The drawing under review shows one solid part. Ordinate dimensions are in mm from its lowest x, y, z. A direction names the side the tool comes from. Coordinates: 2 decimals unless noted, no trailing zeros. Write each loop counter-clockwise with the first axis right and the second up, starting at its lowest first coordinate (ties: lowest second). Pieces come first, ordered by that corner, then holes. Notation, with made-up numbers: (-30.75, 20) -> (-7.75, 20) arc R10 cw to (-7.75, 27) -> close; hole circle Ø7 at (40, 58). An arc over 180 degrees is marked (long way). Put each result on its own line as item: value. Start each with the question number.
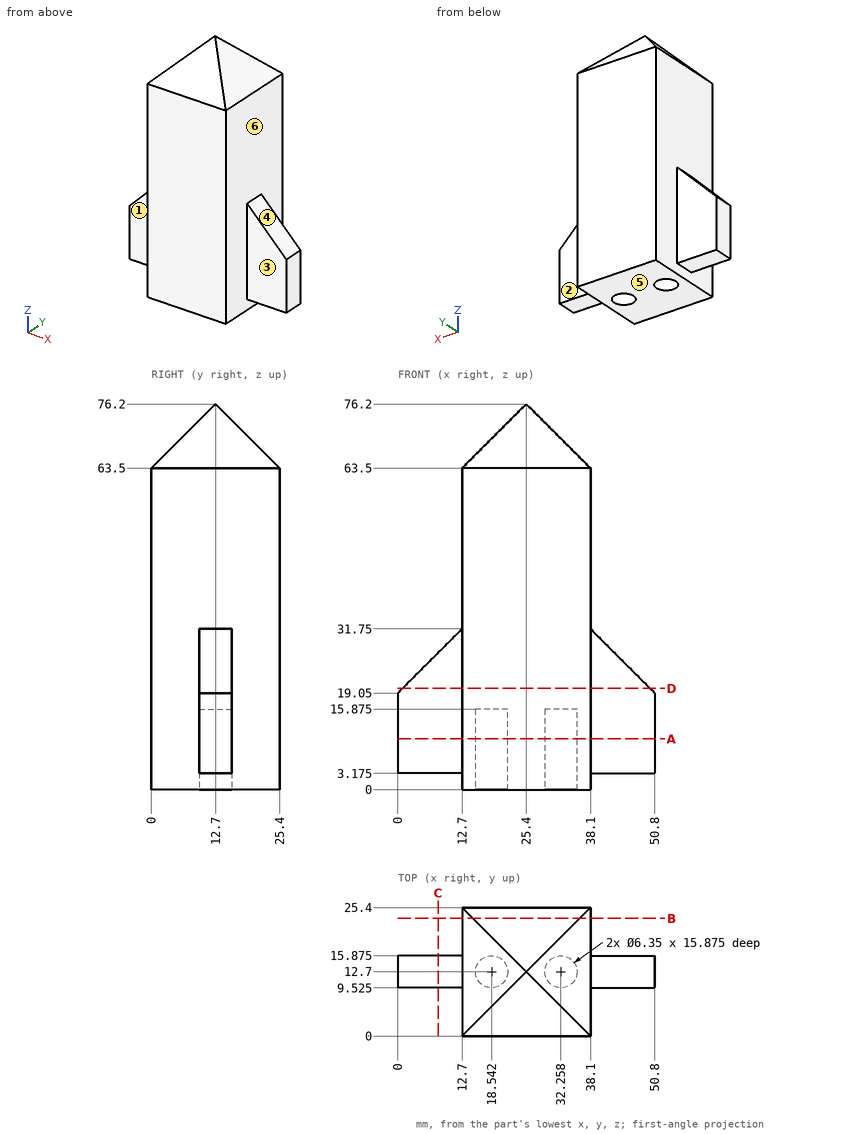
1. The part is to be moulded in two halves that separate along Z. For the marked faces 4, 5 and 6, say which applies: released by +Z, released by -Z, zero draft, split by the parting line, or undercut.
2. Consider section B-B on y = 23.25. State the section outline as (x, z) points.
3. Consider section D-D on z = 20. State the section outline as (x, y) points (3 decimals), then the cut area to 3 significant figures.
4. Tool access review of the marked faces 1, 2 and 3: name each direction out of +Z, -Z, +X, -X, +Y, -Y from which nothing blocks a thin tool from reaching the whole face with its end or side.
5. Consider section A-A on z = 10. State the section outline as (x, y) points (3 decimals), then the cut area to 3 significant figures.
6. Insertion check: P1, Ø3, axis at x = 8, y = 15.5, coming from the -Z side (3 decimals); P2, Ø3, axis at y = 20.5, z = 12, coming from the -X side; P3, Ø5, axis at y = 14, z = 43.5, coming from the +X side; P4, Ø10, axis at x = 18.542, y = 12.7, coming from the -Z side. Each pin has a flat end and moves straight along its axis. Give the tip position at first contact, or say it passes through.
7. Consider section C-C on x = 8. State the section outline as (y, z) points (3 decimals), then the cut area to 3 significant figures.
8. Wall thickness on line 1 (X direction, y = 7.5, z = 8.5); line 2 (Y direction, x = 11.5, z = 20.5) (3 decimals); line 3 (Z direction, x = 21, y = 12) (3 decimals): over which ranges is each line inside the solid? List them lowest first. Write a range as from..to.
Output values:
1. face 4: released by +Z
1. face 5: released by -Z
1. face 6: zero draft
2. outline: (12.7, 0) -> (38.1, 0) -> (38.1, 63.5) -> (35.95, 65.65) -> (14.85, 65.65) -> (12.7, 63.5) -> close
3. outline: (0.95, 9.525) -> (12.7, 9.525) -> (12.7, 0) -> (38.1, 0) -> (38.1, 9.525) -> (49.85, 9.525) -> (49.85, 15.875) -> (38.1, 15.875) -> (38.1, 25.4) -> (12.7, 25.4) -> (12.7, 15.875) -> (0.95, 15.875) -> close
3. area: 794 mm^2
4. face 1: +Z, -Z, -X, -Y
4. face 2: +Z, -Z, +X, +Y
4. face 3: +Z, -Z, +X, -Y
5. outline: (0, 9.525) -> (12.7, 9.525) -> (12.7, 0) -> (38.1, 0) -> (38.1, 9.525) -> (50.8, 9.525) -> (50.8, 15.875) -> (38.1, 15.875) -> (38.1, 25.4) -> (12.7, 25.4) -> (12.7, 15.875) -> (0, 15.875) -> close; hole circle Ø6.35 at (18.542, 12.7); hole circle Ø6.35 at (32.258, 12.7)
5. area: 743 mm^2
6. P1: stops at z = 3.175
6. P2: stops at x = 12.7
6. P3: stops at x = 38.1
6. P4: stops at z = 0
7. outline: (9.525, 3.175) -> (15.875, 3.175) -> (15.875, 27.05) -> (9.525, 27.05) -> close
7. area: 152 mm^2
8. line 1: x = 12.7..38.1
8. line 2: y = 9.525..15.875
8. line 3: z = 15.875..71.8
